from build123d import *

# Parameters (mm, degrees)
ESQUISSE1_R        = 1.5
BOSS_EXTRU_3_DEPTH = 6


with BuildPart() as part:
    # Esquisse1 → Boss.-Extru.3 (new body)
    with BuildSketch(Plane.XY):
        with BuildLine():
            Line((29.100926589, 7.727116755), (19.492495604, 22.948090903))
            Line((19.492495604, 22.948090903), (9.344755552, 16.543141892))
            ThreePointArc((9.344755552, 16.543141892), (-16.066583823, -10.142232706), (18.954034468, 1.320824515))
            Line((18.954034468, 1.320824515), (29.100926589, 7.727116755))
        make_face()
        with Locations((-0.546712729, 15.490355231)):
            Circle(ESQUISSE1_R, mode=Mode.SUBTRACT)
        with Locations((-13.14168478, -8.218644727)):
            Circle(ESQUISSE1_R, mode=Mode.SUBTRACT)
        with Locations((13.688397508, -7.271710504)):
            Circle(ESQUISSE1_R, mode=Mode.SUBTRACT)
        with BuildLine():
            ThreePointArc((-3.468577117, 13.56351624), (-0.423261467, 11.992533082), (2.503723019, 13.774301109))
            ThreePointArc((2.503723019, 13.774301109), (11.869908833, 7.423292012), (13.480638187, -3.777882222))
            ThreePointArc((13.480638187, -3.777882222), (10.597469039, -5.629711358), (10.677033171, -9.055438293))
            ThreePointArc((10.677033171, -9.055438293), (0.493805045, -13.991288596), (-10.01206107, -9.785634018))
            ThreePointArc((-10.01206107, -9.785634018), (-10.174207571, -6.362821724), (-13.180756189, -4.718862816))
            ThreePointArc((-13.180756189, -4.718862816), (-12.363713879, 6.567996584), (-3.468577117, 13.56351624))
        make_face(mode=Mode.SUBTRACT)
    extrude(amount=BOSS_EXTRU_3_DEPTH)


solid = part.part
The listing builds one solid part. Answer for the finished solid, in the listing's coordinates (mm). A direction names the side the tool comes from. Round coordinates to 2 decimals unless told otherwise and drop trailing zeros. Order: outer loops, then holes, each group sorted by start corner. A loop starts at its lowest first (then second) coordinate and runs counter-clockwise, first axis right, second up. Notation, with made-up numbers: (12.5, 69.5) -> (65.5, 69.5) arc R14 ccw to (65.5, 74.5) -> close; hole circle Ø8 at (-21.5, -21.75). An arc over 180 degrees is marked (long way). Write each question's results on one line, items separated by ' | '. Start each with the question number.
Q1. Straight lines are drawn through the part: probe 1 along Y at (x, z) = (-1, 2.25); probe 2 along Y at (x, z) = (11, 3.25); probe 3 along Y at (x, z) = (6.5, 0.6). For each, find the intervals that lie inside material, in ascending order. Write a range as from..to.
Q2. The mould has two halves that part along X. Classify faces 1 (the flat face through (14, 4, 6)), 2 (the cylindrical face through (10.62, -5.59, 2.96)), 3 (the flat face through (23.96, 4.48, 2.96)), 4 (the cylindrical face through (-12.44, 6.42, 2.96)): pulls with the +X half, pulls with the -X half, needs draft (parallel to the pull), parting line crosses it, or undercut.
Q3. Find section B-B (x = 11.5). Determine the outline of the cut face in (y, z), then the cut area to 3 significant figures.
Q4. Find section A-A (y = 0). Determine the outline of the cut face in (x, z), then the cut area to 3 significant figures.
Q5. Find section C-C (z = 2.2). Determine the outline of the cut face in (x, y), then the cut area to 3 significant figures.
Q6. Find section D-D (x = 0). Determine the outline of the cut face in (y, z).
Q7. Which of the six approach directions +Z, -Z, +X, -X, +Y, -Y give full straight-line access (tool end or side, diameter ignored) to faces 5 (the flat face through (14.49, 19.79, 2.96)), 6 (the flat face through (14, 4, 0)), 7 (the cylindrical face through (11.783, 7.561, 2.958))?
Q8. Each of these flat-tipped pins is pushed along its axis until it touches: pin 1 (3 mm diameter, centred on y = -12.5, z = 4.5, fed in from +X); pin 2 (1 mm diameter, centred on x = 14.5, z = 4, fed in from -Y); pin 3 (1 mm diameter, centred on y = -0.5, z = 1, fed in from +X). Where does it stop, or does it pass through?
Worked answers:
1) probe 1: y = -18.97..-13.96, 12.02..14.06, 16.92..18.97 | probe 2: y = -15.49..-5.03, 8.66..17.59 | probe 3: y = -17.85..-12.4, 12.4..17.85
2) face 1: needs draft | face 2: undercut | face 3: pulls with the +X half | face 4: undercut
3) outline: (-15.12, 0) -> (-4.54, 0) -> (-4.54, 6) -> (-15.12, 6) -> close; (7.98, 0) -> (17.9, 0) -> (17.9, 6) -> (7.98, 6) -> close | area: 123 mm2
4) outline: (-19, 0) -> (-14, 0) -> (-14, 6) -> (-19, 6) -> close; (14, 0) -> (19, 0) -> (19, 6) -> (14, 6) -> close | area: 60.0 mm2
5) outline: (9.34, 16.54) arc R19 ccw (long way) to (18.95, 1.32) -> (29.1, 7.73) -> (19.49, 22.95) -> close; hole circle Ø3 at (-13.14, -8.22); hole (-13.18, -4.72) arc R3.5 cw to (-10.01, -9.79) arc R14 ccw to (10.68, -9.06) arc R3.5 cw to (13.48, -3.78) arc R14 ccw to (2.5, 13.77) arc R3.5 cw to (-3.47, 13.56) arc R14 ccw to start; hole circle Ø3 at (-0.55, 15.49); hole circle Ø3 at (13.69, -7.27) | area: 711 mm2
6) outline: (-19, 0) -> (-14, 0) -> (-14, 6) -> (-19, 6) -> close; (12.03, 0) -> (14.09, 0) -> (14.09, 6) -> (12.03, 6) -> close; (16.89, 0) -> (19, 0) -> (19, 6) -> (16.89, 6) -> close
7) face 5: +Z, -Z, +Y | face 6: -Z, +X, -X, +Y, -Y | face 7: +Z, -Z
8) pin 1: stops at x = 15.49 | pin 2: stops at y = -12.85 | pin 3: stops at x = 19
